The listing builds one solid part. Answer for the finished solid, in the listing's coordinates (mm). Face numbers are marked on the shaded views. A direction names the side the tool comes from. Round coordinates to 2 decimals unless told otherwise and drop trailing zeros. Write each loop counter-clockwise with the first axis right and the second up, starting at its lowest first coordinate (ties: lowest second). Pieces come first, ordered by that corner, then holes. Notation, with made-up numbers: (-19.75, 87) - (-1.75, 87) arc R20 ccw to (-1.75, 115) - close; hole circle Ø11 at (-18, 50.5). An arc over 180 degrees is marked (long way). Answer in a Markdown table with one row per item.
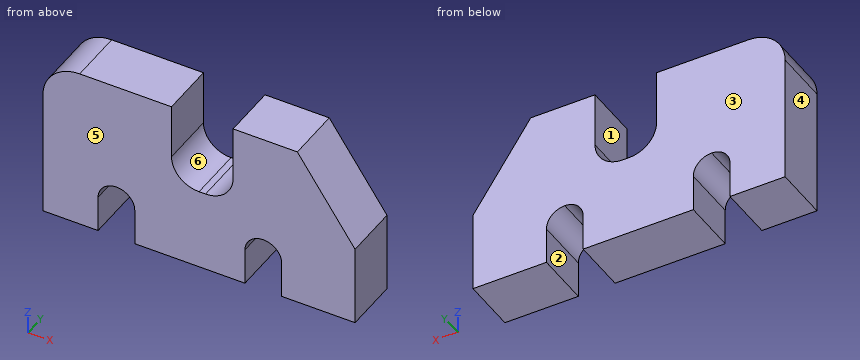
from build123d import *

# Parameters (mm, degrees)
F1_DEPTH = 30


with BuildPart() as f1:
    # F0 (on Front) → F1 (new body)
    with BuildSketch(Plane.XZ):
        with BuildLine():
            Line((-82.660393, 34.991289), (-82.660393, -35.008711))
            Line((-82.660393, -35.008711), (-52.660393, -35.008711))
            Line((-52.660393, -35.008711), (-52.660393, -15.008711))
            ThreePointArc((-52.660393, -15.008711), (-49.731461, -7.937643), (-42.660393, -5.008711))
            ThreePointArc((-42.660393, -5.008711), (-35.589325, -7.937643), (-32.660393, -15.008711))
            Line((-32.660393, -15.008711), (-32.660393, -35.008711))
            Line((-32.660393, -35.008711), (27.339607, -35.008711))
            Line((27.339607, -35.008711), (27.339607, -15.008711))
            ThreePointArc((27.339607, -15.008711), (30.268539, -7.937643), (37.339607, -5.008711))
            ThreePointArc((37.339607, -5.008711), (44.410675, -7.937643), (47.339607, -15.008711))
            Line((47.339607, -15.008711), (47.339607, -35.008711))
            Line((47.339607, -35.008711), (87.339607, -35.008711))
            Line((87.339607, -35.008711), (87.339607, 8.991289))
            Line((87.339607, 8.991289), (55.892236, 54.991289))
            Line((55.892236, 54.991289), (20.892236, 54.991289))
            Line((20.892236, 54.991289), (20.892236, 24.991289))
            ThreePointArc((20.892236, 24.991289), (16.498838, 14.384687), (5.892236, 9.991289))
            Line((5.892236, 9.991289), (2.339607, 9.991289))
            ThreePointArc((2.339607, 9.991289), (-8.266995, 14.384687), (-12.660393, 24.991289))
            Line((-12.660393, 24.991289), (-12.660393, 54.991289))
            Line((-12.660393, 54.991289), (-62.660393, 54.991289))
            ThreePointArc((-62.660393, 54.991289), (-76.802529, 49.133425), (-82.660393, 34.991289))
        make_face()
    extrude(amount=F1_DEPTH)


solid = f1.part
(1) Flat-ended cylindrical pins translate along their axes: pin 1 (1.1 mm diameter, centred on x = 3.5, y = -12, fed in from +Z); pin 2 (9 mm diameter, centred on y = -22, z = 35, fed in from +X); pin 3 (10 mm diameter, centred on y = -22.5, z = 16, fed in from +X). Find the tip coordinate at first contact, or state that the pin passes through.
Checked values:
| item | result |
|---|---|
| pin 1 | stops at z = 9.99 |
| pin 2 | stops at x = 72.64 |
| pin 3 | stops at x = 85.97 |
(2) Section D-D (z = 17.5) is taken. Give the vertices of the cut face in (x, y).
Checked values:
| item | result |
|---|---|
| outline | (-82.66, -30) - (-10.66, -30) - (-10.66, 0) - (-82.66, 0) - close; (18.89, -30) - (81.52, -30) - (81.52, 0) - (18.89, 0) - close |
(3) Find the intervals of material crossed by line 1 (X direction, y = -6.5, z = -25); line 2 (X direction, y = -19.25, z = 26.5); line 3 (X direction, y = -8.75, z = 30), in increasing order.
Checked values:
| item | result |
|---|---|
| line 1 | x = -82.66 to -52.66, -32.66 to 27.34, 47.34 to 87.34 |
| line 2 | x = -82.66 to -12.66, 20.89 to 75.37 |
| line 3 | x = -82.66 to -12.66, 20.89 to 72.98 |
(4) Section C-C (y = -23.75) is taken. Give the vertices of the cut face in (x, z).
Checked values:
| item | result |
|---|---|
| outline | (-82.66, -35.01) - (-52.66, -35.01) - (-52.66, -15.01) arc R10 cw to (-42.66, -5.01) arc R10 cw to (-32.66, -15.01) - (-32.66, -35.01) - (27.34, -35.01) - (27.34, -15.01) arc R10 cw to (37.34, -5.01) arc R10 cw to (47.34, -15.01) - (47.34, -35.01) - (87.34, -35.01) - (87.34, 8.99) - (55.89, 54.99) - (20.89, 54.99) - (20.89, 24.99) arc R15 cw to (5.89, 9.99) - (2.34, 9.99) arc R15 cw to (-12.66, 24.99) - (-12.66, 54.99) - (-62.66, 54.99) arc R20 ccw to (-82.66, 34.99) - close |
(5) Section A-A (z = 49) is taken. Give the vertices of the cut face in (x, y), and give its area (3 significant figures).
Checked values:
| item | result |
|---|---|
| outline | (-76.93, -30) - (-12.66, -30) - (-12.66, 0) - (-76.93, 0) - close; (20.89, -30) - (59.99, -30) - (59.99, 0) - (20.89, 0) - close |
| area | 3,100 mm2 |
(6) For a pull along X with two mould halves and no side action, classify the marked faces 4, 5 and 6 as pulls with the +X half, pulls with the -X half, needs draft (parallel to the pull), parting line crosses it, or undercut.
Checked values:
| item | result |
|---|---|
| face 4 | pulls with the -X half |
| face 5 | needs draft |
| face 6 | undercut |
(7) For the marked faces 1, 2 and 3, determine the directions among +Z, -Z, +X, -X, +Y, -Y from which every point of the face is accessible in a straight line to the end or side of a thin tool.
Checked values:
| item | result |
|---|---|
| face 1 | +Z, +Y, -Y |
| face 2 | -Z, +Y, -Y |
| face 3 | +Z, -Z, +X, -X, +Y |
(8) Section B-B (z = -26) is taken. Give the vertices of the cut face in (x, y).
Checked values:
| item | result |
|---|---|
| outline | (-82.66, -30) - (-52.66, -30) - (-52.66, 0) - (-82.66, 0) - close; (-32.66, -30) - (27.34, -30) - (27.34, 0) - (-32.66, 0) - close; (47.34, -30) - (87.34, -30) - (87.34, 0) - (47.34, 0) - close |
